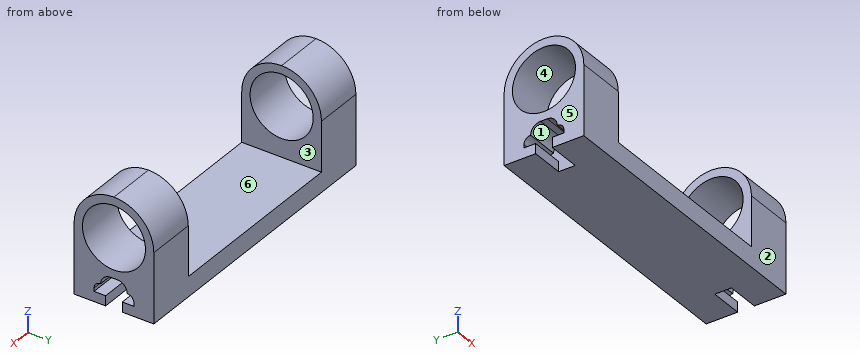
```python
from build123d import *

# Parameters (mm, degrees)
F0_R     = 9.5
F1_DEPTH = 88
F2_W     = 58
F2_H     = 27
F3_DEPTH = 12.5
F4_DEPTH = 10
F6_DEPTH = 10
F7_R     = 2.99999
F8_R     = 1.99999


# Not quite as in the source:
# - a fillet or chamfer is up to 0.001 mm smaller than in the source, because OpenCascade refuses the exact size


with BuildPart() as f1:
    # F0 (on Right) → F1 (new body)
    with BuildSketch(Plane.YZ):
        with BuildLine():
            ThreePointArc((0, 9), (-8.4852813742, 12.5147186258), (-12, 21))
            Line((-12, 21), (-12, 0))
            Line((-12, 0), (-2.5, 0))
            Line((-2.5, 0), (-2.5, 3))
            Line((-2.5, 3), (-6, 3))
            Line((-6, 3), (-6, 6))
            Line((-6, 6), (-4, 6))
            Line((-4, 6), (-4, 9))
            Line((-4, 9), (0, 9))
        make_face()
        Polygon((4, 9), (0, 9), (-4, 9), (-4, 6), (-6, 6), (-6, 3), (-2.5, 3), (-2.5, 0), (2.5, 0), (2.5, 3), (6, 3), (6, 6), (4, 6), align=None)
        with BuildLine():
            Line((12, 0), (12, 21))
            ThreePointArc((12, 21), (8.4852813742, 12.5147186258), (0, 9))
            Line((0, 9), (4, 9))
            Line((4, 9), (4, 6))
            Line((4, 6), (6, 6))
            Line((6, 6), (6, 3))
            Line((6, 3), (2.5, 3))
            Line((2.5, 3), (2.5, 0))
            Line((2.5, 0), (12, 0))
        make_face()
        with BuildLine():
            ThreePointArc((12, 21), (8.4852813742, 29.4852813742), (0, 33))
            ThreePointArc((0, 33), (-8.4852813742, 29.4852813742), (-12, 21))
            ThreePointArc((-12, 21), (-8.4852813742, 12.5147186258), (0, 9))
            ThreePointArc((0, 9), (8.4852813742, 12.5147186258), (12, 21))
        make_face()
        with Locations((0, 21)):
            Circle(F0_R, mode=Mode.SUBTRACT)
    extrude(amount=-F1_DEPTH)

    # F2 (on Front) → F3 (cut, symmetric)
    with BuildSketch(Plane.XZ):
        with Locations((-44, 19.5)):
            Rectangle(F2_W, F2_H)
    extrude(amount=F3_DEPTH, both=True, mode=Mode.SUBTRACT)

    # F0 (on Right) → F4 (cut)
    with BuildSketch(Plane.YZ):
        Polygon((4, 9), (0, 9), (-4, 9), (-4, 6), (-6, 6), (-6, 3), (-2.5, 3), (-2.5, 0), (2.5, 0), (2.5, 3), (6, 3), (6, 6), (4, 6), align=None)
    extrude(amount=-F4_DEPTH, mode=Mode.SUBTRACT)

    # F5 (on face) → F6 (cut)
    with BuildSketch(Plane(origin=(-88, 0, 0), x_dir=(0, -1, 0), z_dir=(-1, 0, 0))):
        Polygon((-2.5, 3), (-2.5, 0), (2.5, 0), (2.5, 3), (6, 3), (6, 6), (4, 6), (4, 9), (0, 9), (-4, 9), (-4, 6), (-6, 6), (-6, 3), align=None)
    extrude(amount=-F6_DEPTH, mode=Mode.SUBTRACT)

    # F7 (radius 3 in the source; OpenCascade refuses exactly that, so slightly less here)
    f7_edges = [f1.edges().sort_by_distance(p)[0] for p in [
        (-83, 4, 9),
        (-83, -4, 9),
        (-5, -4, 9),
        (-5, 4, 9),
    ]]
    fillet(f7_edges, radius=F7_R)

    # F8 (radius 2 in the source; OpenCascade refuses exactly that, so slightly less here)
    f8_edges = [f1.edges().sort_by_distance(p)[0] for p in [
        (-83, -6, 6),
        (-83, 6, 6),
        (-5, 6, 6),
        (-5, -6, 6),
    ]]
    fillet(f8_edges, radius=F8_R)


solid = f1.part
```
Design review of the part built by this model. Coordinates are the model's own, in mm. Face numbers are marked on the shaded views. A direction names the side the tool comes from. Coordinates: 2 decimals unless noted, no trailing zeros. Order: outer loops, then holes, each group sorted by start corner. A loop starts at its lowest first (then second) coordinate and runs counter-clockwise, first axis right, second up.
1) Mouldability with a two-part tool opening along X and no side actions: class the marked faces 4, 5 and 6 as +X half, -X half, draft (parallel to the pull), parting line (faces both ways), or undercut.
2) Take a section at C-C, the plane z = 27.5. Give the boundary of the cut face in (x, y), and give its area (3 significant figures).
3) Wall thickness on line 1 along X through (y, z) = (2, 10); line 2 along Z through (x, y) = (-83.25, 0); line 3 along Z through (x, y) = (-77, 0): over which ranges is each line inside the solid? List them lowest first.
4) For the marked faces 1, 2 and 3, list the 3-axis set-ups (+Z, -Z, +X, -X, +Y, -Y) from which the entire face can be reached by the end or side of a thin tool; tool diameter is ignored.
5) Take a section at A-A, the plane x = -74. Give the boundary of the cut face in (y, z).
6) Take a section at B-B, the plane z = 8. Give the boundary of the cut face in (x, y), and give its area (3 significant figures).
7) Take a section at D-D, the plane x = -63. Give the boundary of the cut face in (y, z).
8) Clearance check with flat-ended pins moving along their axes: pin 1 (2 mm diameter, centred on x = -21, y = -6, fed in from +Z); pin 2 (6 mm diameter, centred on x = -78, y = 9, fed in from -Z); pin 3 (1.6 mm diameter, centred on x = -6.5, y = 0.5, fed in from -Z); pin 4 (1 mm diameter, centred on y = 2, z = 28.5, fed in from +X). State where each tip first meets the part, or that it passes through.
Returned:
1. face 4: draft
1. face 5: -X half
1. face 6: undercut
2. outline: (-88, -10.09) - (-73, -10.09) - (-73, -6.93) - (-88, -6.93) - close; (-88, 6.93) - (-73, 6.93) - (-73, 10.09) - (-88, 10.09) - close; (-15, -10.09) - (0, -10.09) - (0, -6.93) - (-15, -6.93) - close; (-15, 6.93) - (0, 6.93) - (0, 10.09) - (-15, 10.09) - close
2. area: 190 mm2
3. line 1: x = -88 to -73, -15 to 0
3. line 2: z = 9 to 11.5, 30.5 to 33
3. line 3: z = 0 to 11.5, 30.5 to 33
4. face 1: -X
4. face 2: +Z, -Z, +X, -X, -Y
4. face 3: +Z, +Y, -Y
5. outline: (-12, 0) - (12, 0) - (12, 21) arc R12 ccw to (-12, 21) - close; hole circle Ø19 at (0, 21)
6. outline: (-88, -12) - (-73, -12) - (-73, 12) - (-88, 12) - (-88, 3.24) - (-78, 3.24) - (-78, -3.24) - (-88, -3.24) - close; (-15, -12) - (0, -12) - (0, -3.24) - (-10, -3.24) - (-10, 3.24) - (0, 3.24) - (0, 12) - (-15, 12) - close
6. area: 591 mm2
7. outline: (-12, 0) - (12, 0) - (12, 6) - (-12, 6) - close
8. pin 1: stops at z = 6
8. pin 2: stops at z = 0
8. pin 3: stops at z = 8.98
8. pin 4: passes through
